The figure shows three views and two pictorial views of one solid part (mm, origin at its lowest corner). Answer the questions. Give positions to 0.01 mm unless a question says otherwise; leave off trailing zeros. Write each loop counter-clockwise with the first axis right and the second up, starting at its lowest first coordinate (ties: lowest second). Pieces come first, ordered by that corner, then holes. Notation, with made-up numbers: (40, -26.5) - (64, -26.5) arc R10 ccw to (64, -12.5) - close; hole circle Ø1 at (-30, 70.5). An arc over 180 degrees is marked (long way). One line per question, with ' | ' between items. Start each with the question number.
1. Find the intervals of material crossed by L1, parallel to Y at x = 19.45, z = 8; L2, parallel to X at y = 7, z = 22; L3, parallel to Y at x = 17, z = 20.5, in increasing order. Write a range as from..to.
2. A cutting plane is placed at D-D (x = 3). Determine the outline of the cut face in (y, z), then the cut area to 3 significant figures.
3. A cutting plane is placed at A-A (y = 21.2). Determine the outline of the cut face in (x, z), then the cut area to 3 significant figures.
4. A cutting plane is placed at C-C (y = 39). Determine the outline of the cut face in (x, z).
5. Given P1, Ø16, axis at y = 21, z = 16, coming from the -X side; P2, Ø1.5, axis at x = 2.5, z = 16.5, coming from the -Y side, each flat-ended and moving along its own axis, determine where each tip first touches the part or whether it passes through.
6. A cutting plane is placed at B-B (z = 8). Determine the outline of the cut face in (x, y), then the cut area to 3 significant figures.
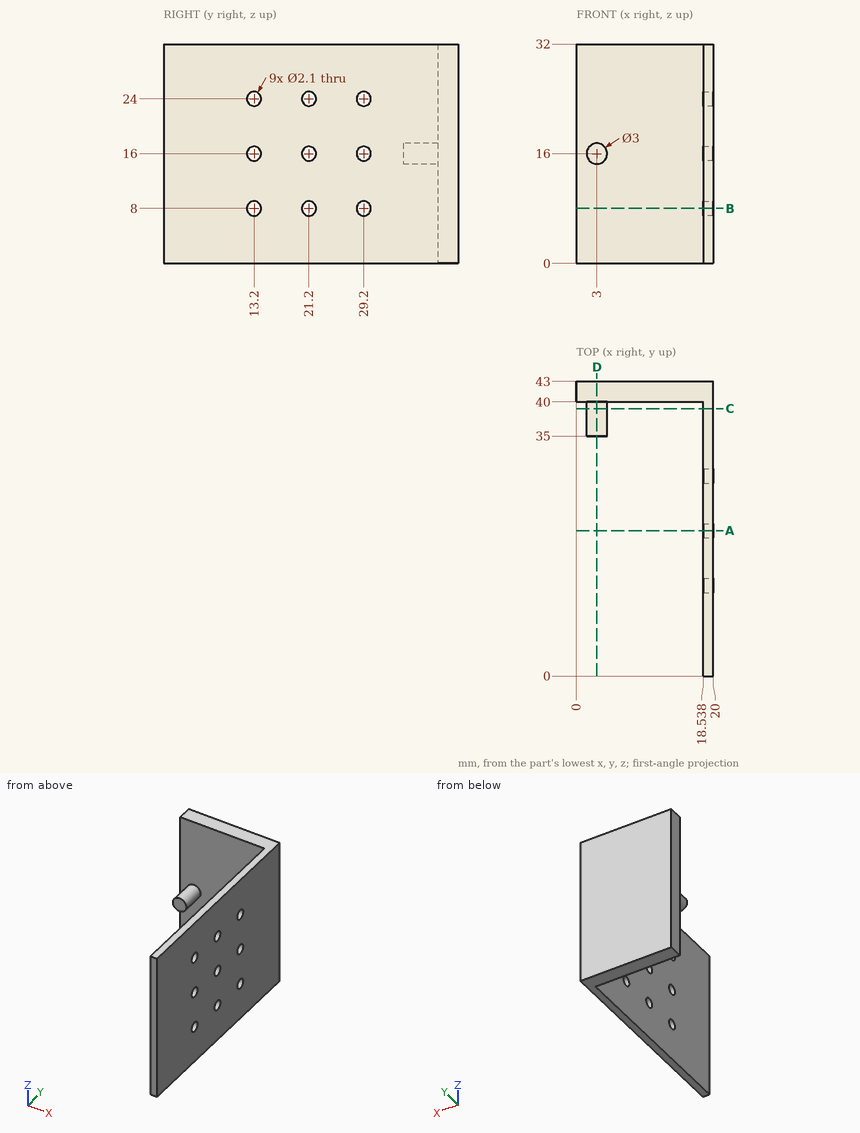
Determined:
1) L1: 0..12.15, 14.25..20.15, 22.25..28.15, 30.25..43 | L2: 18.54..20 | L3: 40..43
2) outline: (35, 14.5) - (40, 14.5) - (40, 0) - (43, 0) - (43, 32) - (40, 32) - (40, 17.5) - (35, 17.5) - close | area: 111 mm2
3) outline: (18.54, 0) - (20, 0) - (20, 6.95) - (18.54, 6.95) - close; (18.54, 9.05) - (20, 9.05) - (20, 14.95) - (18.54, 14.95) - close; (18.54, 17.05) - (20, 17.05) - (20, 22.95) - (18.54, 22.95) - close; (18.54, 25.05) - (20, 25.05) - (20, 32) - (18.54, 32) - close | area: 37.6 mm2
4) outline: circle Ø3 at (3, 16); (18.54, 0) - (20, 0) - (20, 32) - (18.54, 32) - close
5) P1: x = 18.54 | P2: y = 35
6) outline: (0, 40) - (18.54, 40) - (18.54, 30.25) - (20, 30.25) - (20, 43) - (0, 43) - close; (18.54, 0) - (20, 0) - (20, 12.15) - (18.54, 12.15) - close; (18.54, 14.25) - (20, 14.25) - (20, 20.15) - (18.54, 20.15) - close; (18.54, 22.25) - (20, 22.25) - (20, 28.15) - (18.54, 28.15) - close | area: 109 mm2
